Source: CAD feature listing. Evaluate the final solid. Frame: model axes, mm. A direction names the side the tool comes from. Coordinates: 2 decimals unless noted, no trailing zeros. Loops run counter-clockwise (first coordinate to the right, second up) from the corner with the lowest first, then second, coordinate; pieces in that order, holes last.
```python
from build123d import *

# Parameters (mm, degrees)
SKETCH1_W           = 35
SKETCH1_H           = 51
SKETCH1_R           = 2
BOSS_EXTRUDE1_DEPTH = 10
CUT_EXTRUDE4_DEPTH  = 5
CUT_EXTRUDE5_DEPTH  = 33.503845926


with BuildPart() as part:
    # Sketch1 → Boss-Extrude1 (new body)
    with BuildSketch(Plane(origin=(0, 0, 0), x_dir=(1, 0, 0), z_dir=(0, 1, 0))):
        Rectangle(SKETCH1_W, SKETCH1_H)
        with Locations(Location((-12.5, 12.5, 0), (0, 0, 270))):
            Circle(SKETCH1_R, mode=Mode.SUBTRACT)
        with Locations(Location((12.5, 12.5, 0), (0, 0, 90))):
            Circle(SKETCH1_R, mode=Mode.SUBTRACT)
        with Locations(Location((12.5, -12.5, 0), (0, 0, 270))):
            Circle(SKETCH1_R, mode=Mode.SUBTRACT)
        with Locations(Location((-12.5, -12.5, 0), (0, 0, 90))):
            Circle(SKETCH1_R, mode=Mode.SUBTRACT)
        with Locations(Location((0, 22, 0), (0, 0, 270))):
            Circle(SKETCH1_R, mode=Mode.SUBTRACT)
        with Locations(Location((0, -22, 0), (0, 0, 90))):
            Circle(SKETCH1_R, mode=Mode.SUBTRACT)
    extrude(amount=BOSS_EXTRUDE1_DEPTH)

    # Sketch2 → Cut-Extrude4 (cut)
    with BuildSketch(Plane(origin=(0, 0, 0), x_dir=(1, 0, 0), z_dir=(0, 1, 0))):
        Polygon((4.041451884, 22), (2.020725942, 25.5), (-2.020725942, 25.5), (-4.041451884, 22), (-2.020725942, 18.5), (2.020725942, 18.5), align=None)
        Polygon((4.041451884, -22), (2.020725942, -18.5), (-2.020725942, -18.5), (-4.041451884, -22), (-2.020725942, -25.5), (2.020725942, -25.5), align=None)
    extrude(amount=CUT_EXTRUDE4_DEPTH, mode=Mode.SUBTRACT)

    # Sketch4 → Cut-Extrude5 (cut, through all)
    with BuildSketch(Plane(origin=(0, 0, 0), x_dir=(1, 0, 0), z_dir=(0, 1, 0))):
        Polygon((-7.5, 25.5), (-17.5, 15.5), (-17.5, 25.5), align=None)
        Polygon((17.5, -15.5), (7.5, -25.5), (17.5, -25.5), align=None)
    extrude(amount=CUT_EXTRUDE5_DEPTH, mode=Mode.SUBTRACT)


solid = part.part
```
Q1. Section query D-D on y = 8.25. Return the cut outline in (x, z).
Q2. Reachability of faces 1 (the flat face through (0, 2, 18.5)), 2 (the flat face through (-12, 5, -21)), 3 (the flat face through (3.045, 2.465, -23.726)) from +Z, -Z, +X, -X, +Y, -Y: full face, straight path, thin tool, end or side. Return the list, or none.
Q3. Draft query along Z for faces 4 (the flat face through (0, 10, 0)), 5 (the cylindrical face through (11.148, 4.93, -11.026)), 6 (the flat face through (0, 2, -18.5)). Return one class per face: released by +Z, released by -Z, zero draft, split by the parting line, or undercut.
Q4. Material intervals for line 1 along X through (y, z) = (6, 12.5); line 2 along X through (y, z) = (6, -14); line 3 along Z through (x, y) = (-12, 2.75), sorted ascending.
Q5. Section query C-C on z = 13.5. Return the cut outline in (x, y), then the cut area to 3 significant figures.
Q6. Section query B-B on y = 4. Return the cut outline in (x, z).
Q7. First-contact query: pin 1 Ø2 at (x, z) = (-1.5, -22.5) entering from -Y. Flat tip, straight axial feed; report the tip coordinate or a pass-through.
Q8. Section query A-A on x = -12.5. Return the cut outline in (y, z).
Resolved:
1. outline: (-17.5, -15.5) - (-7.5, -25.5) - (17.5, -25.5) - (17.5, 15.5) - (7.5, 25.5) - (-17.5, 25.5) - close; hole circle Ø4 at (-12.5, -12.5); hole circle Ø4 at (-12.5, 12.5); hole circle Ø4 at (0, -22); hole circle Ø4 at (0, 22); hole circle Ø4 at (12.5, -12.5); hole circle Ø4 at (12.5, 12.5)
2. face 1: +Z, -Y
2. face 2: -Z, -X, +Y, -Y
2. face 3: -Y
3. face 4: zero draft
3. face 5: undercut
3. face 6: released by -Z
4. line 1: x = -17.5 to -14.5, -10.5 to 10.5, 14.5 to 17.5
4. line 2: x = -17.5 to -13.82, -11.18 to 11.18, 13.82 to 17.5
4. line 3: z = -21 to -14.44, -10.56 to 10.56, 14.44 to 25.5
5. outline: (-17.5, 0) - (-14.23, 0) - (-14.23, 10) - (-17.5, 10) - close; (-10.77, 0) - (10.77, 0) - (10.77, 10) - (-10.77, 10) - close; (14.23, 0) - (17.5, 0) - (17.5, 10) - (14.23, 10) - close
5. area: 281 mm2
6. outline: (-17.5, -15.5) - (-7.5, -25.5) - (-2.02, -25.5) - (-4.04, -22) - (-2.02, -18.5) - (2.02, -18.5) - (4.04, -22) - (2.02, -25.5) - (17.5, -25.5) - (17.5, 15.5) - (7.5, 25.5) - (2.02, 25.5) - (4.04, 22) - (2.02, 18.5) - (-2.02, 18.5) - (-4.04, 22) - (-2.02, 25.5) - (-17.5, 25.5) - close; hole circle Ø4 at (-12.5, -12.5); hole circle Ø4 at (-12.5, 12.5); hole circle Ø4 at (12.5, -12.5); hole circle Ø4 at (12.5, 12.5)
7. pin 1: stops at y = 5
8. outline: (0, -20.5) - (10, -20.5) - (10, -14.5) - (0, -14.5) - close; (0, -10.5) - (10, -10.5) - (10, 10.5) - (0, 10.5) - close; (0, 14.5) - (10, 14.5) - (10, 25.5) - (0, 25.5) - close
